CAD build for the part. Positions are in the model's coordinates, mm. A direction names the side the tool comes from. Coordinates: 2 decimals unless noted, no trailing zeros. Loops run counter-clockwise (first coordinate to the right, second up) from the corner with the lowest first, then second, coordinate; pieces in that order, holes last. Notation, with made-up numbers: (-30.75, -38.5) -> (-2.75, -38.5) arc R14 cw to (-2.75, -14.5) -> close; hole circle Ø11 at (28, 28). An arc over 180 degrees is marked (long way). Write each question's results on one line, items separated by ' | '.
Autodesk Inventor part; units mm, degrees
ref_plane "YZ Plane" through (0, 0, 0) normal (1, 0, 0) x (0, 1, 0)
ref_plane "XZ Plane" through (0, 0, 0) normal (0, 1, 0) x (-1, 0, 0)
ref_plane "XY Plane" through (0, 0, 0) normal (0, 0, 1) x (1, 0, 0)
sketch "Boceto1" plane through (0, 0, 0) normal (0, 0, 1) x (1, 0, 0)
  line L0 (0, 0) -> (50, 0)
  line L1 (50, 0) -> (50, 68)
  line L2 (50, 68) -> (0, 68)
  line L3 (0, 68) -> (0, 0)
  dimension "d0" = 50
  dimension "d1" = 68
extrude "Extrusión1" add sketch "Boceto1" along normal blind 2
hole "Hole1" at (2.0897, 65.5, 2) direction (0, 0, -1) diameter 3 end through all
hole "Hole2" at (47.5, 65.5, 2) direction (0, 0, -1) diameter 3 end through all
hole "Hole3" at (2.5, 2.5, 2) direction (0, 0, -1) diameter 3 end through all
hole "Hole4" at (47.5, 2.5, 2) direction (0, 0, -1) diameter 3 end through all
fillet "Empalme1" radius 3 1 edges at (50, 68, 1)
fillet "Empalme2" radius 3 1 edges at (0, 68, 1)
fillet "Empalme3" radius 3 1 edges at (0, 0, 1)
fillet "Empalme4" radius 3 1 edges at (50, 0, 1)
sketch "Boceto2" plane through (0, 0, 2) normal (0, 0, 1) x (1, 0, 0)
  line L0 (3, 68) -> (47, 68)
  line L1 (6, 68) -> (6, 60)
  line L2 (6, 60) -> (14, 60)
  line L3 (14, 60) -> (14, 68)
  line L4 (47, 0) -> (3, 0)
  line L5 (6, 68) -> (6, 73)
  line L6 (6, 73) -> (14, 73)
  line L7 (14, 73) -> (14, 68)
  point P0 (0, 0)
  dimension "d47" = 8
  dimension "d48" = 8
  dimension "d49" = 8
  dimension "d63" = 5
extrude "Extrusión2" add sketch "Boceto2" along normal blind 6
sketch "Boceto3" plane through (0, 0, 8) normal (0, 0, 1) x (1, 0, 0)
  line L0 (6, 60) -> (6, 73)
  line L1 (14, 60) -> (6, 60)
  line L2 (14, 73) -> (14, 60)
  line L3 (6, 60) -> (7, 60)
  line L4 (7, 61.5) -> (6, 61.5)
  line L5 (7, 61.5) -> (7, 60)
  line L6 (14, 60) -> (13, 60)
  line L7 (13, 61.5) -> (14, 61.5)
  line L8 (13, 61.5) -> (13, 60)
  line L9 (7, 61.5) -> (13, 61.5)
  point P0 (14, 68)
  point P1 (6, 68)
  point P2 (0, 0)
extrude "Extrusión3" cut sketch "Boceto3" against normal blind 6 contours L5 L9 L8 L1
sketch "Boceto4" plane through (0, 0, 2) normal (0, 0, 1) x (1, 0, 0)
  line L0 (14, 68) -> (14, 60)
  line L1 (6, 60) -> (6, 68)
  line L2 (3, 68) -> (47, 68)
  line L3 (6, 68) -> (14, 68)
  line L4 (21, 68) -> (21, 59)
  line L5 (21, 59) -> (29, 59)
  line L6 (29, 59) -> (29, 68)
  line L7 (21, 68) -> (29, 68)
  point P0 (0, 0)
  dimension "d55" = 8
extrude "Extrusión4" add sketch "Boceto4" along normal blind 4
sketch "Boceto5" plane through (0, 0, 2) normal (0, 0, 1) x (1, 0, 0)
  line L0 (29, 68) -> (47, 68)
  line L1 (50, 68) -> (44, 68)
  line L2 (44, 68) -> (44, 60)
  line L3 (44, 60) -> (36, 60)
  line L4 (36, 60) -> (36, 73)
  line L5 (44, 73) -> (44, 65.5)
  line L6 (44, 73) -> (36, 73)
  point P0 (0, 0)
  dimension "d58" = 6
  dimension "d59" = 8
  dimension "d60" = 13
extrude "Extrusión5" add sketch "Boceto5" along normal blind 6
sketch "Boceto6" plane through (0, 0, 8) normal (0, 0, 1) x (1, 0, 0)
  line L0 (44, 60) -> (36, 60)
  line L1 (37, 61.5) -> (37, 60)
  line L2 (43, 61.5) -> (43, 60)
  line L3 (43, 61.5) -> (37, 61.5)
  line L4 (37, 61.5) -> (37, 60)
  line L5 (43, 60.1438) -> (43, 61.5)
  line L6 (37, 60) -> (43, 60)
  point P0 (0, 0)
extrude "Extrusión6" cut sketch "Boceto6" against normal blind 6
sketch "Boceto7" plane through (0, 0, 2) normal (0, 0, 1) x (1, 0, 0)
  line L0 (0, 3) -> (0, 65)
  line L1 (47, 0) -> (3, 0)
  line L2 (7, 0) -> (7, -1)
  line L3 (7, -1) -> (22, -1)
  line L4 (22, -1) -> (22, 13)
  line L5 (22, 13) -> (7, 13)
  line L6 (7, 13) -> (7, 0)
  point P0 (0, 0)
extrude "Extrusión7" add sketch "Boceto7" along normal blind 5
sketch "Boceto8" plane through (0, 0, 2) normal (0, 0, 1) x (1, 0, 0)
  line L0 (47, 0) -> (22, 0)
  line L1 (35, 0) -> (35, 5)
  line L2 (35, 5) -> (25, 5)
  line L3 (25, 5) -> (25, 0)
  line L4 (35, 0) -> (25, 0)
  point P0 (0, 0)
  dimension "d74" = 5
extrude "Extrusión8" add sketch "Boceto8" along normal blind 3
sketch "Boceto9" plane through (3, 0, 0) normal (0, -1, 0) x (1, 0, 0)
  line L0 (29, 5) -> (22, 5)
  line L1 (32, 5) -> (29, 5)
  line L2 (29, 5) -> (29, 3.7)
  line L3 (29, 3.7) -> (27.7, 3.7)
  line L4 (27.7, 3.7) -> (27.7, 5)
  line L5 (29, 5) -> (27.7, 5)
  point P0 (-3, 0)
  dimension "d78" = 1.3
  dimension "d79" = 1.3
extrude "Extrusión9" add sketch "Boceto9" along normal blind 2
sketch "Boceto10" plane through (0, 0, 2) normal (0, 0, 1) x (1, 0, 0)
  line L0 (50, 65) -> (50, 3)
  line L1 (50, 49) -> (46, 49)
  line L2 (46, 49) -> (46, 43)
  line L3 (46, 43) -> (50, 43)
  line L4 (50, 49) -> (50, 43)
  point P0 (0, 0)
  dimension "d83" = 6
extrude "Extrusión10" add sketch "Boceto10" along normal blind 4
sketch "Boceto11" plane through (50, 65, 2) normal (1, 0, 0) x (0, 0, -1)
  line L0 (-3, -17) -> (-1, -17)
  line L1 (-1, -17) -> (-1, -21)
  line L2 (-1, -21) -> (-3, -21)
  line L3 (-3, -21) -> (-3, -17)
  point P0 (2, -65)
extrude "Extrusión11" add sketch "Boceto11" along normal blind 1
sketch "Boceto12" plane through (0, 0, 2) normal (0, 0, 1) x (1, 0, 0)
  line L0 (47, 0) -> (35, 0)
  line L1 (43, 18) -> (43, 21)
  line L2 (43, 21) -> (37, 21)
  line L3 (37, 21) -> (37, 18)
  line L4 (37, 18) -> (43, 18)
  point P0 (0, 0)
  dimension "d90" = 3
  dimension "d91" = 6
extrude "Extrusión12" add sketch "Boceto12" along normal blind 1
sketch "Boceto13" plane through (0, 0, 5) normal (0, 0, 1) x (1, 0, 0)
  line L0 (35, 5) -> (35, 0)
  line L1 (30.7, 0) -> (25, 0)
  line L2 (32, 0) -> (32, -2)
  line L3 (25, 5) -> (35, 5)
  line L4 (35, 0) -> (25, 0)
  line L5 (25, 5) -> (25, 0)
  line L6 (35, 5) -> (35, 0)
  point P0 (0, 0)
extrude "Extrusión13" add sketch "Boceto13" against normal blind 6.5
sketch "Boceto14" plane through (0, 0, 7) normal (0, 0, 1) x (1, 0, 0)
  line L0 (7, -1) -> (7, 13)
  line L1 (22, -1) -> (7, -1)
  line L2 (22, 13) -> (22, -1)
  line L3 (7, 13) -> (22, 13)
  line L4 (7, 13) -> (22, 13)
  line L5 (22, -1) -> (7, -1)
  point P0 (0, 0)
extrude "Extrusión14" add sketch "Boceto14" against normal blind 8.5
sketch "Boceto15" plane through (0, 0, 6) normal (0, 0, 1) x (1, 0, 0)
  line L0 (50, 49) -> (50, 43)
  line L1 (46, 49) -> (50, 49)
  line L2 (46, 49) -> (50, 49)
  line L3 (50, 43) -> (46, 43)
  line L4 (46, 43) -> (46, 49)
  point P0 (0, 0)
extrude "Extrusión15" add sketch "Boceto15" against normal blind 7.5
properties part number "lipoRiderPro"
1) Drill centre lines: L1, parallel to X at y = 63.5, z = 5; L2, parallel to Y at x = 2.5, z = 1.05; L3, parallel to Y at x = 47.5, z = 1.1. Where is each one in solid material? Low to high. Write a range as from..to.
Outcome:
L1: x = 6..14, 21..29, 36..44 | L2: y = 0.04..1, 4..64.06, 66.94..67.96 | L3: y = 0.04..1, 4..64, 67..67.96
2) Slice it at B-B (y = 33). Write the cut outline in (x, z).
Outcome:
outline: (0, 0) -> (50, 0) -> (50, 2) -> (0, 2) -> close
3) Two-plate mould, pull along X, no slides. Class faces 1 (the cylindrical face through (0.9, 67.14, 1.01)), 2 (the flat face through (37, 61, 5)), 3 (the flat face through (48, 46, 6)): pulls with the +X half, pulls with the -X half, needs draft (parallel to the pull), parting line crosses it, or undercut.
Outcome:
face 1: pulls with the -X half | face 2: undercut | face 3: needs draft
4) Pin check, flat tips, straight feed: pin 1 (3 mm diameter, centred on x = 14, z = 5, fed in from -Y); pin 2 (2 mm diameter, centred on x = 31, z = 2.5, fed in from -Y); pin 3 (3 mm diameter, centred on y = 46, z = 5.5, fed in from +X); pin 4 (3.5 mm diameter, centred on y = 3.5, z = 3, fed in from +X). Stop position of each tip, or through.
Outcome:
pin 1: stops at y = -1 | pin 2: stops at y = 0 | pin 3: stops at x = 51 | pin 4: stops at x = 50
5) Which spindle directions (+Z, -Z, +X, -X, +Y, -Y) get a long thin tool onto all of the face, cutting with end or side? Do faces 4 (the flat face through (40, 71, 2)), 5 (the flat face through (35, 2, 3)), 6 (the flat face through (5, 0, 1)). Say none if no direction does.
Outcome:
face 4: -Z, +X, -X, +Y | face 5: +Z, +X, +Y, -Y | face 6: +Z, -Z, -X, -Y
6) Slice it at A-A (x = 9). Write the cut outline in (y, z), then the cut area to 3 significant figures.
Outcome:
outline: (-1, -1.5) -> (13, -1.5) -> (13, 0) -> (68, 0) -> (68, 2) -> (73, 2) -> (73, 8) -> (61.5, 8) -> (61.5, 2) -> (13, 2) -> (13, 7) -> (-1, 7) -> close | area: 298 mm^2
